```python
from build123d import *

# Parameters (mm, degrees)
BOSS_EXTRUDE1_DEPTH      = 6
BOSS_EXTRUDE1_DEPTH_BACK = 6
SKETCH2_W                = 6.2
SKETCH2_H                = 6.2
CUT_EXTRUDE1_DEPTH       = 3.25
SKETCH3_W                = 6.2
SKETCH3_H                = 6.2
CUT_EXTRUDE2_DEPTH       = 3.25
SKETCH4_W                = 6.2
SKETCH4_H                = 6.2
CUT_EXTRUDE3_DEPTH       = 3.25
FILLET1_R                = 5
SKETCH5_W                = 6.2
SKETCH5_H                = 6.2
CUT_EXTRUDE4_DEPTH       = 38.489999943
SKETCH6_W                = 6.2
SKETCH6_H                = 6.2
CUT_EXTRUDE5_DEPTH       = 32.982302651


with BuildPart() as part:
    # Sketch1 → Boss-Extrude1 (new, two sides: drawn at the far end of the back side and taken through both)
    with BuildSketch(Plane.XY.offset(-BOSS_EXTRUDE1_DEPTH_BACK)):
        Polygon((5.901614565, 38.174412444), (2.949595544, 21.432680643), (6.39642268, 20.824912021), (7.264663568, 25.748950786), (36.808896158, 20.539505456), (35.94065527, 15.615466691), (37.910270776, 15.268170336), (41.040910113, 21.981848059), (41.040910113, 25.981848059), (27.040910113, 32.510155273), align=None)
    extrude(amount=BOSS_EXTRUDE1_DEPTH + BOSS_EXTRUDE1_DEPTH_BACK)

    # Sketch2 → Cut-Extrude1 (cut)
    with BuildSketch(Plane(origin=(4.622386329, 26.214855554, 0), x_dir=(0.9848077530122067, -0.17364817766693813, 0), z_dir=(-0.17364817766693813, -0.9848077530122067, 0))):
        with Locations((8.183038624, 0)):
            Rectangle(SKETCH2_W, SKETCH2_H)
        with Locations((23.183038624, 0)):
            Rectangle(SKETCH2_W, SKETCH2_H)
    extrude(amount=-CUT_EXTRUDE1_DEPTH, mode=Mode.SUBTRACT)

    # Sketch3 → Cut-Extrude2 (cut)
    with BuildSketch(Plane(origin=(9.938936325, 37.092615339, 0), x_dir=(0.9659258262890682, -0.25881904510252135, 0), z_dir=(0.2588190451025213, 0.9659258262890681, 0))):
        with Locations((4.820256949, 0)):
            Rectangle(SKETCH3_W, SKETCH3_H)
    extrude(amount=-CUT_EXTRUDE2_DEPTH, mode=Mode.SUBTRACT)

    # Sketch4 → Cut-Extrude3 (cut)
    with BuildSketch(Plane(origin=(17.281785965, 37.0609096, 0), x_dir=(0.9063077870366484, -0.42261826174070294, 0), z_dir=(0.42261826174070294, 0.9063077870366484, 0))):
        with Locations((16.768002093, 0)):
            Rectangle(SKETCH4_W, SKETCH4_H)
    extrude(amount=-CUT_EXTRUDE3_DEPTH, mode=Mode.SUBTRACT)

    # Fillet1
    fillet1_edges = [part.edges().sort_by_distance(p)[0] for p in [
        (39.475590445, 18.625009197, -6),
        (41.040910113, 23.981848059, -6),
        (39.475590445, 18.625009197, 6),
        (41.040910113, 23.981848059, 6),
    ]]
    fillet(fillet1_edges, radius=FILLET1_R)

    # Sketch5 → Cut-Extrude4 (cut, through all)
    with BuildSketch(Plane(origin=(9.097774429, 33.953356403, 0), x_dir=(0.9659258262890683, -0.2588190451025211, 0), z_dir=(0.2588190451025211, 0.9659258262890683, 0))):
        with Locations((4.820256949, 0)):
            Rectangle(SKETCH5_W, SKETCH5_H)
    extrude(amount=-CUT_EXTRUDE4_DEPTH, mode=Mode.SUBTRACT)

    # Sketch6 → Cut-Extrude5 (cut, through all)
    with BuildSketch(Plane(origin=(15.908276614, 34.115409292, 0), x_dir=(0.9063077870366483, -0.42261826174070316, 0), z_dir=(0.42261826174070316, 0.9063077870366483, 0))):
        with Locations((16.768002093, 0)):
            Rectangle(SKETCH6_W, SKETCH6_H)
    extrude(amount=-CUT_EXTRUDE5_DEPTH, mode=Mode.SUBTRACT)


solid = part.part
```
For this review, take the finished solid that the model builds, in its own axes (mm). A direction names the side the tool comes from. Give positions to 0.01 mm unless a question says otherwise; leave off trailing zeros. Order: outer loops, then holes, each group sorted by start corner. A loop starts at its lowest first (then second) coordinate and runs counter-clockwise, first axis right, second up.
1) Take a section at B-B (y = 23.75). Give the boundary of the cut face in (x, z).
2) Take a section at D-D (y = 26.5). Give the boundary of the cut face in (x, z), then the cut area to 3 significant figures.
3) Take a section at C-C (x = 31). Give the boundary of the cut face in (y, z), then the cut area to 3 significant figures.
4) Take a section at A-A (z = 0). Give the boundary of the cut face in (x, y).
5) For faces 1 (the face through (30, 26, -3.1)), 2 (the face through (25.97, 25.75, 0.04)), 3 (the face through (33.62, 25.09, 0.04)), list the 3-axis set-ups (+Z, -Z, +X, -X, +Y, -Y) from which the entire face can be reached by the end or side of a thin tool; tool diameter is ignored.
6) The part is to be moulded in two halves that separate along Y. For faces 4 (the face through (10.13, 31.16, 0.04)), 5 (the face through (16.01, 25.83, -0.04)), 6 (the face through (4.446, 29.921, -0.084)), 7 (the face through (41.041, 24, 0)), say which applies: released by +Y, released by -Y, zero draft, split by the parting line, or undercut.
7) Wall thickness on line 1 (X direction, y = 25, z = 2); line 2 (X direction, y = 28.5, z = 0); line 3 (Z direction, x = 32.5, y = 25): over which ranges is each line inside the solid? List them lowest first.
8) Insertion check: pin 1 (4 mm diameter, centred on x = 35.5, z = 4.5, fed in from -Y); pin 2 (2 mm diameter, centred on x = 33, z = -3.5, fed in from -Y); pin 3 (1.5 mm diameter, centred on x = 22.5, z = -2, fed in from -Y); pin 4 (1 mm diameter, centred on x = 28, y = 20, fed in from -Z). Each pin has a flat end and moves straight along its axis. Give the tip position at first contact, or say it passes through.
Derived:
1. outline: (3.36, -6) - (6.91, -6) - (6.91, 6) - (3.36, 6) - close; (18.6, -6) - (36.04, -6) arc R5 ccw to (41.04, -1) - (41.04, 1) arc R5 ccw to (36.04, 6) - (18.6, 6) - close; hole (24.58, -3.1) - (33, -3.1) - (33, 3.1) - (24.58, 3.1) - close
2. outline: (3.84, -6) - (36.04, -6) arc R5 ccw to (39.93, -4.14) - (39.93, 4.14) arc R5 ccw to (36.04, 6) - (3.84, 6) - close; hole (8.88, -3.1) - (16.13, -3.1) - (16.13, 3.1) - (8.88, 3.1) - close; hole (27.44, -3.1) - (34.28, -3.1) - (34.28, 3.1) - (27.44, 3.1) - close
2. area: 341 mm2
3. outline: (21.56, -6) - (30.66, -6) - (30.66, -3.1) - (21.56, -3.1) - close; (21.56, 3.1) - (30.66, 3.1) - (30.66, 6) - (21.56, 6) - close
3. area: 52.8 mm2
4. outline: (2.95, 21.43) - (6.4, 20.82) - (7.26, 25.75) - (8.62, 25.51) - (11.6, 36.65) - (5.9, 38.17) - close; (15.59, 27.58) - (16.3, 27.46) - (15.73, 24.26) - (24.4, 22.73) - (24.96, 25.93) - (27, 25.57) - (29.67, 31.28) - (27.04, 32.51) - (17.59, 35.04) - close; (31.9, 21.4) - (36.81, 20.54) - (35.94, 15.62) - (37.91, 15.27) - (41.04, 21.98) - (41.04, 25.98) - (35.29, 28.66) - close
5. face 1: none
5. face 2: -Y
5. face 3: +Y
6. face 4: released by -Y
6. face 5: undercut
6. face 6: released by +Y
6. face 7: zero draft
7. line 1: x = 3.58 to 7.13, 15.87 to 24.8, 33.58 to 40.94
7. line 2: x = 4.2 to 9.42, 15.84 to 28.37, 35.21 to 35.64
7. line 3: z = -6 to -3.1, 3.1 to 6
8. pin 1: stops at y = 15.39
8. pin 2: stops at y = 21.03
8. pin 3: stops at y = 22.93
8. pin 4: passes through
